Input: part model. Units: mm. Frame: model coordinates. A direction names the side the tool comes from. Round coordinates to 2 decimals unless told otherwise and drop trailing zeros. Order: outer loops, then holes, each group sorted by start corner. A loop starts at its lowest first (then second) coordinate and runs counter-clockwise, first axis right, second up. Notation, with made-up numbers: (88, 69) -> (140, 69) arc R13 ccw to (140, 79) -> close; hole circle Ø10 at (27.5, 69). An arc over 180 degrees is marked (long way). Use a Markdown table: item, result.
from build123d import *

# Parameters (mm, degrees)
F0_R     = 50.8
F1_DEPTH = 12.7


with BuildPart() as f1:
    # F0 (on Front) → F1 (new body)
    with BuildSketch(Plane.XZ):
        Circle(F0_R)
        with BuildLine():
            ThreePointArc((-6.35, -37.567107), (-38.1, 0), (-6.35, 37.567107))
            Line((-6.35, 37.567107), (-6.35, -37.567107))
        make_face(mode=Mode.SUBTRACT)
        with BuildLine():
            Line((6.35, -37.567107), (6.35, 37.567107))
            ThreePointArc((6.35, 37.567107), (38.1, 0), (6.35, -37.567107))
        make_face(mode=Mode.SUBTRACT)
    extrude(amount=F1_DEPTH)


solid = f1.part
1) Set-up query: faces 5 (the flat face through (-1, 0, 1)), 6 (the flat face through (6.35, -6, -1)). Return all of +Z, -Z, +X, -X, +Y, -Y with unobstructed straight access to the full face (end or side cutting, diameter ignored); none if empty.
Results found:
| item | result |
|---|---|
| face 5 | +Z, -Z, +X, -X, +Y |
| face 6 | +Y, -Y |
2) Line query: L1, parallel to X at y = -3.5, z = 32; L2, parallel to X at y = -11.75, z = -24.5; L3, parallel to Z at x = 11.5, y = -5.25. Output: solid intervals per line, ascending. Write a range as [from, to].
Results found:
| item | result |
|---|---|
| L1 | x = [-39.45, -20.68], [-6.35, 6.35], [20.68, 39.45] |
| L2 | x = [-44.5, -29.18], [-6.35, 6.35], [29.18, 44.5] |
| L3 | z = [-49.48, -36.32], [36.32, 49.48] |
3) Cut plane B-B on x = -27. Return loops of the section in (y, z).
Results found:
| item | result |
|---|---|
| outline | (-12.7, -43.03) -> (0, -43.03) -> (0, -26.88) -> (-12.7, -26.88) -> close; (-12.7, 26.88) -> (0, 26.88) -> (0, 43.03) -> (-12.7, 43.03) -> close |
4) Cut plane C-C on y = -5. Return loops of the section in (x, z), and give its area (3 significant figures).
Results found:
| item | result |
|---|---|
| outline | circle Ø101.6 at (0, 0); hole (-6.35, -37.57) -> (-6.35, 37.57) arc R38.1 ccw to start; hole (6.35, -37.57) arc R38.1 ccw to (6.35, 37.57) -> close |
| area | 4,510 mm² |
5) Pull-direction query (Z, two-part tool) for faces 1 (the flat face through (-1, -12.7, 1)), 2 (the cylindrical face through (-11.012, -6.261, -49.592)), 3 (the cylindrical face through (38.093, -6.261, 0.748)), 4 (the flat face through (-6.35, -6, 1)); classes: +Z half, -Z half, draft (parallel to the pull), parting line (faces both ways), or undercut.
Results found:
| item | result |
|---|---|
| face 1 | draft |
| face 2 | parting line |
| face 3 | undercut |
| face 4 | undercut |
6) Cut plane A-A on z = 0. Return loops of the section in (x, y), and give its area (3 significant figures).
Results found:
| item | result |
|---|---|
| outline | (-50.8, -12.7) -> (-38.1, -12.7) -> (-38.1, 0) -> (-50.8, 0) -> close; (-6.35, -12.7) -> (6.35, -12.7) -> (6.35, 0) -> (-6.35, 0) -> close; (38.1, -12.7) -> (50.8, -12.7) -> (50.8, 0) -> (38.1, 0) -> close |
| area | 484 mm² |
7) Cut plane D-D on z = 35.5. Return loops of the section in (x, y).
Results found:
| item | result |
|---|---|
| outline | (-36.34, -12.7) -> (-13.83, -12.7) -> (-13.83, 0) -> (-36.34, 0) -> close; (-6.35, -12.7) -> (6.35, -12.7) -> (6.35, 0) -> (-6.35, 0) -> close; (13.83, -12.7) -> (36.34, -12.7) -> (36.34, 0) -> (13.83, 0) -> close |
8) Pin query (flat end, axial travel): pin 1 Ø6 at (x, y) = (22, -2) entering from +Z; pin 2 Ø1 at (y, z) = (-2.5, 28) entering from -X; pin 3 Ø12 at (x, z) = (19, -38.5) entering from +Y; pin 4 Ø12 at (x, z) = (28.5, -14.5) entering from -Y. Return the tip coordinate at first contact, or that it passes through.
Results found:
| item | result |
|---|---|
| pin 1 | stops at z = 47.11 |
| pin 2 | stops at x = -42.71 |
| pin 3 | stops at y = 0 |
| pin 4 | passes through |
